from build123d import *

# Parameters (mm, degrees)
SKETCH1_W               = 30
SKETCH1_H               = 50
BOSS_EXTRUDE1_DEPTH     = 50
SKETCH2_W               = 30
SKETCH2_H               = 20
BOSS_EXTRUDE2_DEPTH     = 30
SKETCH3_W               = 30
SKETCH3_H               = 20
CUT_EXTRUDE1_DEPTH      = 10
SKETCH4_W               = 30
SKETCH4_H               = 20
BOSS_EXTRUDE3_DEPTH     = 10
SKETCH6_W               = 30
SKETCH6_H               = 50
CUT_EXTRUDE2_DEPTH      = 10
BOSS_EXTRUDE6_DEPTH     = 30
SKETCH10_W              = 30
SKETCH10_H              = 10
BOSS_EXTRUDE8_DEPTH     = 5
SKETCH11_W              = 30
SKETCH11_H              = 10
BOSS_EXTRUDE9_DEPTH     = 5
BOSS_EXTRUDE10_DEPTH    = 10
BOSS_EXTRUDE11_DEPTH    = 10
SKETCH14_W              = 30
SKETCH14_H              = 10
CUT_EXTRUDE3_DEPTH      = 30
CUT_EXTRUDE3_DEPTH_BACK = 30
CUT_EXTRUDE4_DEPTH      = 20
SKETCH19_W              = 36.844767133
SKETCH19_H              = 14.176927822
BOSS_EXTRUDE18_DEPTH    = 10
SKETCH20_W              = 30
SKETCH20_H              = 10
BOSS_EXTRUDE19_DEPTH    = 10
SKETCH22_W              = 36.844767133
SKETCH22_H              = 14.176927822
CUT_EXTRUDE6_DEPTH      = 9.75
SKETCH25_W              = 36.844767133
SKETCH25_H              = 14.176927822
CUT_EXTRUDE14_DEPTH     = 0.12
SKETCH26_W              = 36.844767133
SKETCH26_H              = 14.176927822
CUT_EXTRUDE15_DEPTH     = 0.12
SKETCH29_W              = 36.844767133
SKETCH29_H              = 14.176927822
BOSS_EXTRUDE21_DEPTH    = 0.05
SKETCH31_W              = 60
SKETCH31_H              = 30
BOSS_EXTRUDE25_DEPTH    = 0.08
SKETCH32_W              = 30
SKETCH32_H              = 10
CUT_EXTRUDE22_DEPTH     = 10
SKETCH38_W              = 10
SKETCH38_H              = 9.92
CUT_EXTRUDE26_DEPTH     = 0.001
SKETCH39_W              = 30
SKETCH39_H              = 10
BOSS_EXTRUDE31_DEPTH    = 0.001


with BuildPart() as part:
    # Sketch1 → Boss-Extrude1 (new body)
    with BuildSketch(Plane.XY):
        with Locations((15, 25)):
            Rectangle(SKETCH1_W, SKETCH1_H)
    extrude(amount=BOSS_EXTRUDE1_DEPTH)

    # Sketch2 → Boss-Extrude2 (add)
    with BuildSketch(Plane.XY.offset(50)):
        with Locations((-15, 20)):
            Rectangle(SKETCH2_W, SKETCH2_H)
    extrude(amount=-BOSS_EXTRUDE2_DEPTH)

    # Sketch3 → Cut-Extrude1 (cut)
    with BuildSketch(Plane.XY.offset(50)):
        with Locations((-15, 20)):
            Rectangle(SKETCH3_W, SKETCH3_H)
    extrude(amount=-CUT_EXTRUDE1_DEPTH, mode=Mode.SUBTRACT)

    # Sketch4 → Boss-Extrude3 (add)
    with BuildSketch(Plane(origin=(0, 0, 20), x_dir=(-1, 0, 0), z_dir=(0, 0, -1))):
        with Locations((15, 20)):
            Rectangle(SKETCH4_W, SKETCH4_H)
    extrude(amount=BOSS_EXTRUDE3_DEPTH)

    # Sketch6 → Cut-Extrude2 (cut)
    with BuildSketch(Plane(origin=(0, 50, 0), x_dir=(1, 0, 0), z_dir=(0, 1, 0))):
        with Locations((15, -25)):
            Rectangle(SKETCH6_W, SKETCH6_H)
    extrude(amount=-CUT_EXTRUDE2_DEPTH, mode=Mode.SUBTRACT)

    # Sketch9 → Boss-Extrude6 (add)
    with BuildSketch(Plane.XY.offset(30)):
        Polygon((-30, 0), (0, 0), (0, 40), align=None)
    extrude(amount=-BOSS_EXTRUDE6_DEPTH)

    # Sketch10 → Boss-Extrude8 (add)
    with BuildSketch(Plane.XY.offset(50)):
        with Locations((15, 45)):
            Rectangle(SKETCH10_W, SKETCH10_H)
    extrude(amount=-BOSS_EXTRUDE8_DEPTH)

    # Sketch11 → Boss-Extrude9 (add)
    with BuildSketch(Plane(origin=(0, 0, 45), x_dir=(-1, 0, 0), z_dir=(0, 0, -1))):
        with Locations((-15, 45)):
            Rectangle(SKETCH11_W, SKETCH11_H)
    extrude(amount=BOSS_EXTRUDE9_DEPTH)

    # Sketch12 → Boss-Extrude10 (add)
    with BuildSketch(Plane(origin=(0, 40, 0), x_dir=(1, 0, 0), z_dir=(0, 1, 0))):
        Polygon((0, -40), (30, -30), (30, -40), align=None)
    extrude(amount=BOSS_EXTRUDE10_DEPTH)

    # Sketch13 → Boss-Extrude11 (add)
    with BuildSketch(Plane(origin=(0, 40, 0), x_dir=(1, 0, 0), z_dir=(0, 1, 0))):
        Polygon((0, 0), (30, 0), (30, -20), (0, -10), align=None)
    extrude(amount=BOSS_EXTRUDE11_DEPTH)

    # Sketch14 → Cut-Extrude3 (cut, two sides)
    with BuildSketch(Plane(origin=(0, 0, 0), x_dir=(0, 0, -1), z_dir=(1, 0, 0))) as cut_extrude3_sk:
        with Locations((-25, 5)):
            Rectangle(SKETCH14_W, SKETCH14_H)
    extrude(amount=CUT_EXTRUDE3_DEPTH, mode=Mode.SUBTRACT)
    extrude(cut_extrude3_sk.sketch, amount=-CUT_EXTRUDE3_DEPTH_BACK, mode=Mode.SUBTRACT)

    # Sketch15 → Cut-Extrude4 (cut)
    with BuildSketch(Plane.XY.offset(30)):
        Polygon((-7.5, 30), (0, 30), (0, 40), align=None)
    extrude(amount=-CUT_EXTRUDE4_DEPTH, mode=Mode.SUBTRACT)

    # Sketch19 → Boss-Extrude18 (add)
    with BuildSketch(Plane(origin=(0, 10, 0), x_dir=(-1, 0, 0), z_dir=(0, -1, 0))):
        with Locations((11.577616434, -32.911536089)):
            Rectangle(SKETCH19_W, SKETCH19_H)
    extrude(amount=BOSS_EXTRUDE18_DEPTH)

    # Sketch20 → Boss-Extrude19 (add)
    with BuildSketch(Plane.XY.offset(50)):
        with Locations((-15, 5)):
            Rectangle(SKETCH20_W, SKETCH20_H)
    extrude(amount=-BOSS_EXTRUDE19_DEPTH)

    # Sketch22 → Cut-Extrude6 (cut)
    with BuildSketch(Plane(origin=(0, 0, 0), x_dir=(-1, 0, 0), z_dir=(0, -1, 0))):
        with Locations((11.577616434, -32.911536089)):
            Rectangle(SKETCH22_W, SKETCH22_H)
    extrude(amount=-CUT_EXTRUDE6_DEPTH, mode=Mode.SUBTRACT)

    # Sketch25 → Cut-Extrude14 (cut)
    with BuildSketch(Plane(origin=(0, 9.75, 0), x_dir=(-1, 0, 0), z_dir=(0, -1, 0))):
        with Locations((11.577616434, -32.911536089)):
            Rectangle(SKETCH25_W, SKETCH25_H)
    extrude(amount=-CUT_EXTRUDE14_DEPTH, mode=Mode.SUBTRACT)

    # Sketch26 → Cut-Extrude15 (cut)
    with BuildSketch(Plane.XZ.offset(-9.87)):
        with Locations((-11.577616434, 32.911536089)):
            Rectangle(SKETCH26_W, SKETCH26_H)
    extrude(amount=-CUT_EXTRUDE15_DEPTH, mode=Mode.SUBTRACT)

    # Sketch29 → Boss-Extrude21 (add)
    with BuildSketch(Plane.XZ.offset(-10)):
        with Locations((-11.577616434, 32.911536089)):
            Rectangle(SKETCH29_W, SKETCH29_H)
    extrude(amount=BOSS_EXTRUDE21_DEPTH)

    # Sketch31 → Boss-Extrude25 (add)
    with BuildSketch(Plane(origin=(0, 10, 0), x_dir=(-1, 0, 0), z_dir=(0, -1, 0))):
        with Locations((0, -25)):
            Rectangle(SKETCH31_W, SKETCH31_H)
    extrude(amount=BOSS_EXTRUDE25_DEPTH)

    # Sketch32 → Cut-Extrude22 (cut)
    with BuildSketch(Plane.XY.offset(50)):
        with Locations((-15, 5)):
            Rectangle(SKETCH32_W, SKETCH32_H)
    extrude(amount=-CUT_EXTRUDE22_DEPTH, mode=Mode.SUBTRACT)

    # Sketch38 → Cut-Extrude26 (cut)
    with BuildSketch(Plane.ZY):
        with Locations((45, 4.96)):
            Rectangle(SKETCH38_W, SKETCH38_H)
    extrude(amount=-CUT_EXTRUDE26_DEPTH, mode=Mode.SUBTRACT)

    # Sketch39 → Boss-Extrude31 (add)
    with BuildSketch(Plane(origin=(0, 0, 0), x_dir=(-1, 0, 0), z_dir=(0, -1, 0))):
        with Locations((14.999, -45)):
            Rectangle(SKETCH39_W, SKETCH39_H)
    extrude(amount=-BOSS_EXTRUDE31_DEPTH)


solid = part.part
For this review, take the finished solid that the model builds, in its own axes (mm). A direction names the side the tool comes from. Round coordinates to 2 decimals unless told otherwise and drop trailing zeros. Loops run counter-clockwise (first coordinate to the right, second up) from the corner with the lowest first, then second, coordinate; pieces in that order, holes last. Notation, with made-up numbers: (34, -37) - (81, -37) arc R11 ccw to (81, -31) - close; hole circle Ø1 at (88.5, 73). An arc over 180 degrees is marked (long way). Use one line per item in the form item = value.
1) Mouldability with a two-part tool opening along Z and no side actions: class faces 4 (the face through (15, 45, 15)), 5 (the face through (-21, 22, 10)), 6 (the face through (0.001, 5, 45)) as pulls with the +Z half, pulls with the -Z half, needs draft (parallel to the pull), parting line crosses it, or undercut.
Solutions:
face_4 = undercut
face_5 = pulls with the -Z half
face_6 = needs draft
2) Clearance check with flat-ended pins moving along their axes: P1, Ø1.5, axis at x = -20, y = 20.5, coming from the -Z side; P2, Ø2, axis at x = -5, y = 37, coming from the +Z side; P3, Ø3, axis at x = -2, z = 29.5, coming from the +Y side; P4, Ø10, axis at x = -21, y = 19.5, coming from the +Z side. State where each tip first meets the part, or that it passes through.
Solutions:
P1 = 10
P2 = through
P3 = 30
P4 = 40
3) We need section A-A on x = -25. State how many separate pieces and enclosed holes the cut face has, then the cut area to 3 significant figures.
Solutions:
separate_pieces = 3
enclosed_holes = 0
area = 669 mm2
4) We need section C-C on z = 37. Write out the cut boundary in (x, y).
Solutions:
outline = (-30, 9.92) - (30, 9.92) - (30, 50) - (9, 50) - (9, 40) - (0, 40) - (0, 30) - (-30, 30) - close
5) We need section D-D on x = 6. Write out the cut boundary in (y, z), then the cut area to 3 significant figures.
Solutions:
outline = (0, 0) - (50, 0) - (50, 12) - (40, 12) - (40, 38) - (50, 38) - (50, 50) - (0, 50) - (0, 40) - (9.92, 40) - (9.92, 10) - (0, 10) - close
area = 1,940 mm2
6) We need section B-B on y = 20. Write out the cut boundary in (x, z), then the cut area to 3 significant figures.
Solutions:
outline = (-30, 10) - (-15, 10) - (-15, 0) - (30, 0) - (30, 50) - (0, 50) - (0, 40) - (-30, 40) - close
area = 2,550 mm2
7) Tool access review of faces 1 (the face through (14, 5, 40)), 2 (the face through (-2, 33, 10)), 3 (the face through (0, 45, 5)): name each direction out of +Z, -Z, +X, -X, +Y, -Y from which nothing blocks a thin tool from reaching the whole face with its end or side.
Solutions:
face_1 = +X, -X, -Y
face_2 = +Z, -X, +Y
face_3 = +Z, -Z, -X, +Y
8) Wall thickness on probe 1 along Z at (x, y) = (27, 7); probe 2 along Z at (x, y) = (-16.5, 14.5); probe 3 along Y at (x, z) = (19, 30): over which ranges is each line inside the solid? List them lowest first.
Solutions:
probe_1 = 0 to 10, 40 to 50
probe_2 = 0 to 40
probe_3 = 9.92 to 40
